```python
from build123d import *

# Parameters (mm, degrees)
F0_R     = 15
F1_DEPTH = 10
F3_D     = 6


# Not quite as in the source:
# - a feature names something its author has since deleted; it is built from what else it names


with BuildPart() as f1:
    # F0 (on Front) → F1 (new body)
    with BuildSketch(Plane.XZ):
        with BuildLine():
            Line((-125, -10), (-125, -20))
            Line((-125, -20), (-78, -20))
            Line((-78, -20), (-78, -19))
            ThreePointArc((-78, -19), (-76.5355339059, -15.4644660941), (-73, -14))
            Line((-73, -14), (73, -14))
            ThreePointArc((73, -14), (76.5355339059, -15.4644660941), (78, -19))
            Line((78, -19), (78, -20))
            Line((78, -20), (125, -20))
            Line((125, -20), (125, -10))
            ThreePointArc((125, -10), (122.0710678119, -2.9289321881), (115, 0))
            Line((115, 0), (102.1720946881, 0))
            ThreePointArc((102.1720946881, 0), (96.3439915213, 1.8739177043), (92.7001654958, 6.7933573047))
            Line((92.7001654958, 6.7933573047), (22.8206678375, 213.2066426953))
            ThreePointArc((22.8206678375, 213.2066426953), (19.176841812, 218.1260822957), (13.3487386452, 220))
            Line((13.3487386452, 220), (0, 220))
            Line((0, 220), (-13.3487386452, 220))
            ThreePointArc((-13.3487386452, 220), (-19.176841812, 218.1260822957), (-22.8206678375, 213.2066426953))
            Line((-22.8206678375, 213.2066426953), (-92.7001654958, 6.7933573047))
            ThreePointArc((-92.7001654958, 6.7933573047), (-96.3439915213, 1.8739177043), (-102.1720946881, 0))
            Line((-102.1720946881, 0), (-115, 0))
            ThreePointArc((-115, 0), (-122.0710678119, -2.9289321881), (-125, -10))
        make_face()
        with BuildLine():
            ThreePointArc((5, 30), (0, 25), (-5, 30))
            Line((-5, 30), (-5, 150))
            ThreePointArc((-5, 150), (0, 155), (5, 150))
            Line((5, 150), (5, 30))
        make_face(mode=Mode.SUBTRACT)
        with Locations((0, 200)):
            Circle(F0_R, mode=Mode.SUBTRACT)
    extrude(amount=F1_DEPTH)

    # F3 (through all)
    with Locations(Plane.XY):
        with Locations((-110, -5), (110, -5)):
            Hole(F3_D / 2)


solid = f1.part
```
Geometry: final body of the model. Coordinates: model frame, mm. A direction names the side the tool comes from. Coordinates: 2 decimals unless noted, no trailing zeros. Order: outer loops, then holes, each group sorted by start corner. A loop starts at its lowest first (then second) coordinate and runs counter-clockwise, first axis right, second up.
Item 1: Section query C-C (z = 90). Output: boundary loops of the cut face in (x, y), then the cut area to 3 significant figures.
Answer:
outline: (-64.53, -10) - (-5, -10) - (-5, 0) - (-64.53, 0) - close; (5, -10) - (64.53, -10) - (64.53, 0) - (5, 0) - close
area: 1,190 mm2
Item 2: Section query D-D (z = 165). Output: boundary loops of the cut face in (x, y), then the cut area to 3 significant figures.
Answer:
outline: (-39.14, -10) - (39.14, -10) - (39.14, 0) - (-39.14, 0) - close
area: 783 mm2
Item 3: Material intervals for line 1 along Z through (x, y) = (0, -7.25); line 2 along Y through (x, z) = (-110, -15.5); line 3 along X through (y, z) = (-8.5, 138.5), sorted ascending.
Answer:
line 1: z = -14 to 25, 155 to 185, 215 to 220
line 2: y = -10 to -8, -2 to 0
line 3: x = -48.11 to -5, 5 to 48.11
Item 4: Contact query for flat-ended pins moving along their axis: P1, Ø5, axis at x = -111.5, y = -4.5, coming from the +Z side; P2, Ø3, axis at y = -5, z = 75.5, coming from the +X side; P3, Ø3, axis at y = -2, z = 101, coming from the -X side. Output: stop coordinate, or through.
Answer:
P1: stops at z = 0
P2: stops at x = 69.95
P3: stops at x = -61.32
Item 5: Draft query along X for faces 1 (the face through (96.415, -4.93, 1.823)), 2 (the face through (107.14, -4.1, -10.14)), 3 (the face through (-19.106, -4.93, 218.177)). Return one class per face: released by +X, released by -X, zero draft, split by the parting line, or undercut.
Answer:
face 1: released by +X
face 2: undercut
face 3: released by -X
Item 6: Access query for faces 4 (the face through (107, -3, 0)), 5 (the face through (-107, -4, 0)), 6 (the face through (-1, -5, -14)), 7 (the face through (-112.86, -4.1, -10.14)), 8 (the face through (0, -5, 25)). Directions: +Z, -Z, +X, -X, +Y, -Y. A direction counts if a zero-diameter tool reaches every point of the face in a straight line with its end or side. Return the directions, or none.
Answer:
face 4: +Z, +X, +Y, -Y
face 5: +Z, -X, +Y, -Y
face 6: -Z, +Y, -Y
face 7: +Z, -Z
face 8: +Y, -Y
Item 7: Section query A-A (y = -5). State how many separate pieces and enclosed holes the cut face has, then the cut area to 3 significant figures.
Answer:
separate pieces: 3
enclosed holes: 2
area: 27,200 mm2
Item 8: Section query B-B (x = -110). Output: boundary loops of the cut face in (y, z), then the cut area to 3 significant figures.
Answer:
outline: (-10, -20) - (-8, -20) - (-8, 0) - (-10, 0) - close; (-2, -20) - (0, -20) - (0, 0) - (-2, 0) - close
area: 80.0 mm2
